Input: part model. Units: mm. Frame: model coordinates. A direction names the side the tool comes from. Coordinates: 2 decimals unless noted, no trailing zeros. Loops run counter-clockwise (first coordinate to the right, second up) from the corner with the lowest first, then second, coordinate; pieces in that order, holes last. Notation, with made-up numbers: (35.25, 40) - (48.25, 40) arc R17 ccw to (48.25, 54) - close; hole circle Ø5 at (-9.5, 1.5). An arc over 180 degrees is marked (long way). Use one line per item in the form item = value.
from build123d import *

# Parameters (mm, degrees)
F0_R     = 15.9004
F1_DEPTH = 7.239
F2_R     = 1.89865
F3_DEPTH = 14.479


with BuildPart() as f1:
    # F0 (on Top) → F1 (new body, symmetric)
    with BuildSketch(Plane.XY):
        Circle(F0_R)
    extrude(amount=F1_DEPTH, both=True)

    # F2 (on face) → F3 (cut, through all)
    with BuildSketch(Plane.XY.offset(7.239)):
        Circle(F2_R)
    extrude(amount=-F3_DEPTH, mode=Mode.SUBTRACT)

    # F4 (on Right) → F5 (revolve, cut)
    with BuildSketch(Plane.YZ):
        Polygon((20.401963, -4.7117), (20.401963, 4.7117), (12.3317, 4.7117), (7.62, 0), (12.3317, -4.7117), align=None)
        Polygon((11.294965, 9.063118), (4.195787, 9.063118), (4.195787, 1.963941), align=None)
    revolve(axis=Axis((0, 0, 4.896712), (0, 0, 1)), mode=Mode.SUBTRACT)


solid = f1.part
Q1. Cut plane C-C, the plane z = 6.25. Return loops of the section in (x, y), then the cut area to 3 significant figures.
Check values:
outline = circle Ø31.8 at (0, 0); circle Ø8.39 at (0, 0); hole circle Ø16.96 at (0, 0); hole circle Ø3.8 at (0, 0)
area = 612 mm²
Q2. Cut plane D-D, the plane z = -4.25. Return loops of the section in (x, y), then the cut area to 3 significant figures.
Check values:
outline = circle Ø23.74 at (0, 0); hole circle Ø3.8 at (0, 0)
area = 431 mm²
Q3. First-contact query: P1, Ø1, axis at x = 2, z = -2, coming from the +Y side; P2, Ø1, axis at y = 1.5, z = -1.5, coming from the +X side; P3, Ø5, axis at y = -4, z = -4, coming from the -X side; P4, Ø6, axis at x = -5.5, y = 7, coming from the +Z side. Flat tips, straight axial feed; report the tip coordinate or a pass-through.
Check values:
P1 = 9.93
P2 = 9.51
P3 = -15.82
P4 = 7.24
Q4. Set-up query: faces 5 (the flat face through (7, -7, 7.239)), 6 (the flat face through (12, 5, 4.712)), 7 (the cylindrical face through (-3.538, 2.256, 4.565)). Return all of +Z, -Z, +X, -X, +Y, -Y with unobstructed straight access to the full face (end or side cutting, diameter ignored); none if empty.
Check values:
face_5 = +Z, +X, -X, +Y, -Y
face_6 = none
face_7 = +Z
Q5. Cut plane A-A, the plane y = 0. Return loops of the section in (x, z), then the cut area to 3 significant figures.
Check values:
outline = (-15.9, -7.24) - (-1.9, -7.24) - (-1.9, 7.24) - (-4.2, 7.24) - (-4.2, 1.96) - (-9.47, 7.24) - (-15.9, 7.24) - (-15.9, 4.71) - (-12.33, 4.71) - (-7.62, 0) - (-12.33, -4.71) - (-15.9, -4.71) - close; (1.9, -7.24) - (15.9, -7.24) - (15.9, -4.71) - (12.33, -4.71) - (7.62, 0) - (12.33, 4.71) - (15.9, 4.71) - (15.9, 7.24) - (9.47, 7.24) - (4.2, 1.96) - (4.2, 7.24) - (1.9, 7.24) - close
area = 266 mm²
Q6. Ray query, line 1 along Z through (x, y) = (14.5, 2.5); line 2 along Y through (x, z) = (3, 2.75); line 3 along Z through (x, y) = (-7, 7). Return the intervals inside material, ascending. Write a range as [from, to].
Check values:
line_1 = [-7.24, -4.71], [4.71, 7.24]
line_2 = [-9.93, -3.98], [-2.93, 2.93], [3.98, 9.93]
line_3 = [-7.24, -2.28], [2.28, 7.24]
Q7. Pull-direction query (Z, two-part tool) for faces 1 (the flat face through (2, -1, 7.239)), 2 (the cylindrical face through (1.8, 0.6, 0.1)), 3 (the conical face through (7.727, -1.716, -0.295)), 4 (the flat face through (0, -3, -7.239)); classes: pulls with the +Z half, pulls with the -Z half, needs draft (parallel to the pull), parting line crosses it, or undercut.
Check values:
face_1 = pulls with the +Z half
face_2 = needs draft
face_3 = undercut
face_4 = pulls with the -Z half
